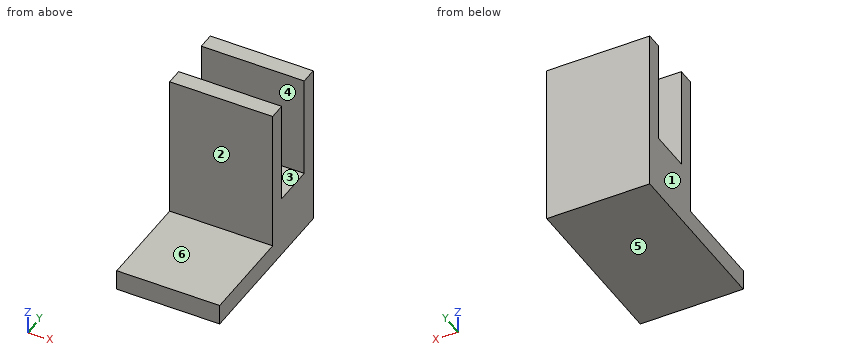
from build123d import *

# Parameters (mm, degrees)
EXTRUDE_1_DEPTH = 12.5


with BuildPart() as part:
    # 草图1 → 凸台-拉伸1 (new, symmetric)
    with BuildSketch(Plane(origin=(0, 0, 0), x_dir=(0, 0, -1), z_dir=(1, 0, 0))):
        Polygon((-40, 14.827740225), (-40, 18.827740225), (0, 18.827740225), (0, 0), (0, -22.636773072), (-5, -22.636773072), (-5, 0.827740225), (-40, 0.827740225), (-40, 4.827740225), (-15, 4.827740225), (-15, 14.827740225), align=None)
    extrude(amount=EXTRUDE_1_DEPTH, both=True)


solid = part.part
The listing builds one solid part. Answer for the finished solid, in the listing's coordinates (mm). Face numbers are marked on the shaded views. A direction names the side the tool comes from. Round coordinates to 2 decimals unless told otherwise and drop trailing zeros. Order: outer loops, then holes, each group sorted by start corner. A loop starts at its lowest first (then second) coordinate and runs counter-clockwise, first axis right, second up. Notation, with made-up numbers: (75, 4.25) -> (118, 4.25) arc R31 cw to (118, 35.25) -> close; hole circle Ø9 at (-5.75, 56.25). An arc over 180 degrees is marked (long way). Write each question's results on one line, items separated by ' | '. Start each with the question number.
Q1. Straight lines are drawn through the part: probe 1 along Y at (x, z) = (-10, 34); probe 2 along Z at (x, y) = (1.5, -16); probe 3 along Z at (x, y) = (0.25, 12). For each, find the intervals that lie inside material, in ascending order. Write a range as from..to.
Q2. Find section D-D (z = 10.5). Determine the outline of the cut face in (x, y).
Q3. The mould has two halves that part along Y. Classify the marked faces 1, 2 and 3: pulls with the +Y half, pulls with the -Y half, needs draft (parallel to the pull), parting line crosses it, or undercut.
Q4. Which of the six approach directions +Z, -Z, +X, -X, +Y, -Y give full straight-line access (tool end or side, diameter ignored) to the marked faces 4, 5 and 6?
Q5. Find section A-A (z = 27). Determine the outline of the cut face in (x, y).
Q6. Find section B-B (x = 8). Determine the outline of the cut face in (y, z).
Q7. Each of these flat-tipped pins is pushed along its axis until it touches: pin 1 (5 mm diameter, centred on x = 5, y = 13, fed in from +Z); pin 2 (7.5 mm diameter, centred on x = 0.5, z = 16, fed in from -Y); pin 3 (7 mm diameter, centred on x = 5, y = -5.5, fed in from +Z). Where does it stop, or does it pass through?
Q8. Find section C-C (y = -20). Determine the outline of the cut face in (x, z), then the cut area to 3 significant figures.
Worked answers:
1) probe 1: y = 0.83..4.83, 14.83..18.83 | probe 2: z = 0..5 | probe 3: z = 0..15
2) outline: (-12.5, 0.83) -> (12.5, 0.83) -> (12.5, 18.83) -> (-12.5, 18.83) -> close
3) face 1: needs draft | face 2: pulls with the -Y half | face 3: undercut
4) face 4: +Z, +X, -X | face 5: -Z, +X, -X, +Y, -Y | face 6: +Z, +X, -X, -Y
5) outline: (-12.5, 0.83) -> (12.5, 0.83) -> (12.5, 4.83) -> (-12.5, 4.83) -> close; (-12.5, 14.83) -> (12.5, 14.83) -> (12.5, 18.83) -> (-12.5, 18.83) -> close
6) outline: (-22.64, 0) -> (18.83, 0) -> (18.83, 40) -> (14.83, 40) -> (14.83, 15) -> (4.83, 15) -> (4.83, 40) -> (0.83, 40) -> (0.83, 5) -> (-22.64, 5) -> close
7) pin 1: stops at z = 40 | pin 2: stops at y = 0.83 | pin 3: stops at z = 5
8) outline: (-12.5, 0) -> (12.5, 0) -> (12.5, 5) -> (-12.5, 5) -> close | area: 125 mm2
